Could you check a few things on this model? Use its own coordinates, in mm. A direction names the side the tool comes from. Coordinates: 2 decimals unless noted, no trailing zeros. Order: outer loops, then holes, each group sorted by start corner. A loop starts at its lowest first (then second) coordinate and runs counter-clockwise, first axis right, second up. Notation, with made-up numbers: (82, 49) -> (122, 49) arc R37 cw to (122, 86) -> close; hole circle Ø10 at (69.25, -3.5). An arc over 180 degrees is marked (long way). Use a Markdown table: item, result. Add a question column.
1) If we section it at B-B (y = 0): Write out the boundary of the cut face in (x, z).
2) Will these pins go through, and if not, where does the flat tip stop? pin 1 Ø6 at (x, y) = (0, 0) entering from +Z; pin 2 Ø5.5 at (x, z) = (21, 1.5) entering from +Y; pin 3 Ø12 at (x, y) = (-5, 18.5) entering from -Z; pin 4 Ø1.5 at (y, z) = (0, -22) entering from -X.
3) If I drill on L1, parallel to Y at x = 0, z = -20.25; L2, parallel to Z at x = 25, y = 2, over which ranges is the centre line in solid material (lowest first)? Write a range as [from, to].
4) If we section it at D-D (x = 25): Write out the boundary of the cut face in (y, z).
5) If we section it at A-A (x = 0): Write out the boundary of the cut face in (y, z), plus the area to 3 significant figures.
6) Which directions (+Z, -Z, +X, -X, +Y, -Y) give clear straight access to the entire face, cutting with the end or side of a thin tool? Please do faces 4 (the flat face through (19, 10, 2)), 5 (the flat face through (0, 3, -25)).
7) Thinking about a two-plate mould opening in X: for faces 1 (the cylindrical face through (6.466, 2.681, -12.325)), 2 (the flat face through (8, -10, 2)), 3 (the cylindrical face through (-0.54, 2.44, -10.21)), which applies, +X half, -X half, draft (parallel to the pull), parting line (faces both ways), or undercut?
8) If we section it at C-C (z = 0.5): Write out the boundary of the cut face in (x, y), plus the area to 3 significant figures.
```python
from build123d import *

# Parameters (mm, degrees)
SKETCH_R     = 2.5
PAD_DEPTH    = 5
FILLET_R     = 3
SKETCH001_R  = 7
PAD001_DEPTH = 25
SKETCH002_R  = 2.5
POCKET_DEPTH = 30.001


with BuildPart() as part:
    # Sketch → Pad (new body)
    with BuildSketch(Plane.XY):
        Polygon((-10, -10), (30, -10), (30, 10), (10, 10), (10, 25), (-10, 25), align=None)
        Circle(SKETCH_R, mode=Mode.SUBTRACT)
    extrude(amount=PAD_DEPTH)

    # Fillet
    fillet_edges = [part.edges().sort_by_distance(p)[0] for p in [
        (30, 10, 2.5),
        (30, -10, 2.5),
    ]]
    fillet(fillet_edges, radius=FILLET_R)

    # Sketch001 → Pad001 (new body)
    with BuildSketch(Plane(origin=(0, 0, 0), x_dir=(1, 0, 0), z_dir=(0, 0, -1))):
        Circle(SKETCH001_R)
    extrude(amount=PAD001_DEPTH)

    # Sketch002 → Pocket (cut, through all)
    with BuildSketch(Plane(origin=(0, 0, -25), x_dir=(1, 0, 0), z_dir=(0, 0, -1))):
        Circle(SKETCH002_R)
    extrude(amount=-POCKET_DEPTH, mode=Mode.SUBTRACT)


solid = part.part
```
Answer sheet:
| question | item | result |
|---|---|---|
| 1 | outline | (-10, 0) -> (-7, 0) -> (-7, -25) -> (-2.5, -25) -> (-2.5, 5) -> (-10, 5) -> close; (2.5, -25) -> (7, -25) -> (7, 0) -> (30, 0) -> (30, 5) -> (2.5, 5) -> close |
| 2 | pin 1 | z = 5 |
| 2 | pin 2 | y = 10 |
| 2 | pin 3 | z = 0 |
| 2 | pin 4 | x = -7 |
| 3 | L1 | [-7, -2.5], [2.5, 7] |
| 3 | L2 | [0, 5] |
| 4 | outline | (-10, 0) -> (10, 0) -> (10, 5) -> (-10, 5) -> close |
| 5 | outline | (-10, 0) -> (-7, 0) -> (-7, -25) -> (-2.5, -25) -> (-2.5, 5) -> (-10, 5) -> close; (2.5, -25) -> (7, -25) -> (7, 0) -> (25, 0) -> (25, 5) -> (2.5, 5) -> close |
| 5 | area | 375 mm2 |
| 6 | face 4 | +Z, -Z, +X, +Y |
| 6 | face 5 | -Z, +X, -X, +Y, -Y |
| 7 | face 1 | parting line |
| 7 | face 2 | draft |
| 7 | face 3 | undercut |
| 8 | outline | (-10, -10) -> (27, -10) arc R3 ccw to (30, -7) -> (30, 7) arc R3 ccw to (27, 10) -> (10, 10) -> (10, 25) -> (-10, 25) -> close; hole circle Ø5 at (0, 0) |
| 8 | area | 1,080 mm2 |
